Design review of the part built by this model. Coordinates are the model's own, in mm. A direction names the side the tool comes from. Give positions to 0.01 mm unless a question says otherwise; leave off trailing zeros. Write each loop counter-clockwise with the first axis right and the second up, starting at its lowest first coordinate (ties: lowest second). Pieces come first, ordered by that corner, then holes. Notation, with made-up numbers: M -27.5,-5 L -4.5,-5 A25 cw -4.5,11 Z; hole C 88,14 d3. An arc over 180 degrees is marked long. Use a Markdown table: item, result. Add a question column.
```python
from build123d import *

# Parameters (mm, degrees)
F0_R     = 5.5626
F1_DEPTH = 2.3876
F2_R     = 2.3876
F3_DEPTH = 0.7874
F4_R     = 1.1303
F5_DEPTH = 3.176
F6_SIZE  = 0.254


with BuildPart() as f1:
    # F0 (on Top) → F1 (new body)
    with BuildSketch(Plane.XY):
        Circle(F0_R)
    extrude(amount=F1_DEPTH)

    # F2 (on face) → F3 (join)
    with BuildSketch(Plane.XY.offset(2.3876)):
        Circle(F2_R)
    extrude(amount=F3_DEPTH)

    # F4 (on face) → F5 (cut, through all)
    with BuildSketch(Plane.XY.offset(3.175)):
        Circle(F4_R)
    extrude(amount=-F5_DEPTH, mode=Mode.SUBTRACT)

    # F6
    f6_edges = [f1.edges().sort_by_distance(p)[0] for p in [
        (-5.5626, 0, 2.3876),
        (-5.5626, 0, 0),
    ]]
    chamfer(f6_edges, length=F6_SIZE)


solid = f1.part
```
(1) Add section A-A on x = 0. Give the boundary of the cut face in (y, z) (3 decimals).
(2) Add section D-D on z = 1.95. Give the boundary of the cut face in (x, y), then the cut area to 3 significant figures.
(3) For pin 1 (1.5 mm diameter, centred on y = -3.5, z = 1, fed in from +X); pin 2 (1.5 mm diameter, centred on x = 1, z = 0.5, fed in from +Y), all flat-tipped, find the tip position at first contact; note any pin that passes through.
(4) The part is to be moulded in two halves that separate along Y. For faces 1 (the flat face through (-1.3, 0.1, 0)), 2 (the cylindrical face through (-0.52, -2.33, 2.78)), 3 (the cylindrical face through (-0.245, -1.103, 1.61)), say which applies: released by +Y, released by -Y, zero draft, split by the parting line, or undercut.
(5) Wall thickness on L1, parallel to Y at x = 0, z = 0.7; L2, parallel to Z at x = 2.25, y = -1; L3, parallel to Y at x = -1, z = 0.55: over which ranges is each line inside the solid? List them lowest first.
(6) Machinability: for faces 4 (the cylindrical face through (5.306, 1.671, 1.181)), 5 (the flat face through (1.1, -2.3, 2.388)), which of the approach directions +Z, -Z, +X, -X, +Y, -Y give a long, thin tool a straight path to every point of the face, cutting with its end or side? Answer none if there is none.
(7) Add section C-C on z = 2.75. Give the boundary of the cut face in (x, y).
From the geometry:
| question | item | result |
|---|---|---|
| 1 | outline | M -5.563,0.254 L -5.309,0 L -1.13,0 L -1.13,3.175 L -2.388,3.175 L -2.388,2.388 L -5.309,2.388 L -5.563,2.134 Z; M 1.13,0 L 5.309,0 L 5.563,0.254 L 5.563,2.134 L 5.309,2.388 L 2.388,2.388 L 2.388,3.175 L 1.13,3.175 Z |
| 2 | outline | C 0,0 d11.13; hole C 0,0 d2.26 |
| 2 | area | 93.2 mm^2 |
| 3 | pin 1 | stops at x = 4.84 |
| 3 | pin 2 | stops at y = 5.56 |
| 4 | face 1 | zero draft |
| 4 | face 2 | split by the parting line |
| 4 | face 3 | undercut |
| 5 | L1 | y = -5.56 to -1.13, 1.13 to 5.56 |
| 5 | L2 | z = 0 to 2.39 |
| 5 | L3 | y = -5.47 to -0.53, 0.53 to 5.47 |
| 6 | face 4 | +Z, -Z |
| 6 | face 5 | +Z |
| 7 | outline | C 0,0 d4.78; hole C 0,0 d2.26 |
